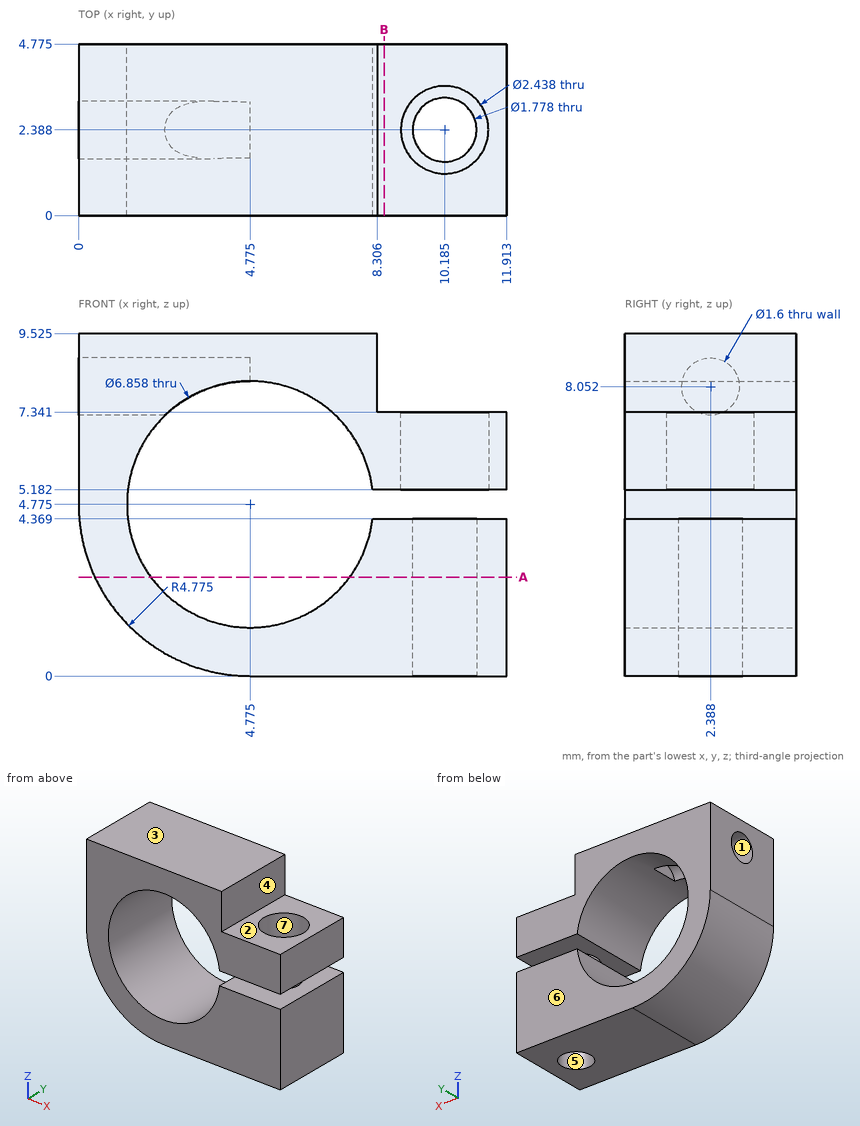
Source: three-view drawing plus pictorial views. Frame: mm from the lowest corner of the part. A direction names the side the tool comes from. Give positions to 0.01 mm unless a question says otherwise; leave off trailing zeros. Order: outer loops, then holes, each group sorted by start corner. A loop starts at its lowest first (then second) coordinate and runs counter-clockwise, first axis right, second up. Notation, with made-up numbers: M 37.5,7 L 69.5,7 A32 ccw 69.5,46 Z; hole C -11.5,51 d1. An arc over 180 degrees is marked long. One line per question, with ' | ' between items. Start each with the question number.
1. Section query A-A (z = 2.75). Count the separate pieces of the cut face and the enclosed holes in it.
2. Section query B-B (x = 8.5). Return the cut outline in (y, z) (1 decimal).
3. Access query for the marked faces 1, 2 and 3. Directions: +Z, -Z, +X, -X, +Y, -Y. A direction counts if a zero-diameter tool reaches every point of the face in a straight line with its end or side. Return the directions, or none.
4. First-contact query: pin 1 Ø1.6 at (x, y) = (10.19, 2.39) entering from +Z; pin 2 Ø1.1 at (x, y) = (9.5, 1.5) entering from +Z; pin 3 Ø1.4 at (y, z) = (2.39, 8.05) entering from -X (1 decimal). Flat tips, straight axial feed; report the tip coordinate or a pass-through.
5. Pull-direction query (X, two-part tool) for the marked faces 4, 5, 6 and 7; classes: released by +X, released by -X, zero draft, split by the parting line, or undercut.
6. Material intervals for probe 1 along Z at (x, y) = (9, 2.8); probe 2 along X at (y, z) = (2.7, 6.75) (1 decimal); probe 3 along X at (y, z) = (3.15, 5.75) (1 decimal), sorted ascending. Write a range as [from, to].
Here are the results:
1) separate pieces: 2 | enclosed holes: 1
2) outline: M 0,0 L 4.8,0 L 4.8,4.4 L 0,4.4 Z; M 0,5.2 L 4.8,5.2 L 4.8,7.3 L 0,7.3 Z
3) face 1: -X | face 2: +Z, +X, +Y, -Y | face 3: +Z, +X, -X, +Y, -Y
4) pin 1: through | pin 2: z = 7.34 | pin 3: x = 4.8
5) face 4: released by +X | face 5: undercut | face 6: zero draft | face 7: undercut
6) probe 1: [0, 4.37], [5.18, 7.34] | probe 2: [0, 2], [7.6, 9], [11.4, 11.9] | probe 3: [0, 1.5], [8.1, 9.2], [11.1, 11.9]
